Input: part model. Units: mm. Frame: model coordinates. A direction names the side the tool comes from. Round coordinates to 2 decimals unless told otherwise and drop trailing zeros. Write each loop counter-clockwise with the first axis right and the second up, starting at its lowest first coordinate (ties: lowest second). Pieces come first, ordered by that corner, then holes. Notation, with made-up numbers: M 22.5,-21 L 44.5,-21 A14 ccw 44.5,-13 Z; hole C 29,89.5 d7. An arc over 180 degrees is marked long. Use one line per item in the form item = value. Start each with the question number.
Autodesk Inventor part; units mm, degrees
ref_plane "YZ Plane" through (0, 0, 0) normal (1, 0, 0) x (0, 1, 0)
ref_plane "XZ Plane" through (0, 0, 0) normal (0, 1, 0) x (-1, 0, 0)
ref_plane "XY Plane" through (0, 0, 0) normal (0, 0, 1) x (1, 0, 0)
sketch "Sketch1" plane through (0, 0, 0) normal (1, 0, 0) x (0, 1, 0)
  line L0 (0, 0) -> (-165.1, 0) construction
  line L1 (-165.1, 0) -> (-165.1, 152.4) construction
  line L2 (-165.1, 152.4) -> (0, 152.4) construction
  line L3 (0, 152.4) -> (0, 0) construction
  line L4 (0, 152.4) -> (-38.1, 152.4)
  line L5 (-165.1, 0) -> (-165.1, 38.1)
  line L6 (-165.1, 38.1) -> (-38.1, 152.4)
  line L7 (0, 152.4) -> (0, 0)
  line L8 (0, 0) -> (-165.1, 0)
  dimension "d0" = 165.1
  dimension "d1" = 152.4
  dimension "d2" = 38.1
  dimension "d3" = 38.1
extrude "Extrusion1" add sketch "Sketch1" along normal blind 6.35
sketch "Sketch2" plane through (0, 0, 0) normal (-1, 0, 0) x (0, 0, 1)
  line L0 (0, -165.1) -> (0, 0)
  line L1 (38.1, -165.1) -> (0, -165.1)
  point P0 (25.4, -139.7)
  point P1 (25.4, -88.9)
  point P2 (25.4, -38.1)
  dimension "d6" = 25.4
  dimension "d7" = 25.4
  dimension "d8" = 25.4
  dimension "d9" = 25.4
  dimension "d10" = 50.8
  dimension "d11" = 50.8
hole "Hole1" at (0, -139.7, 25.4) at (0, -88.9, 25.4) at (0, -38.1, 25.4) direction (1, 0, 0) diameter 6.35 end through all
sketch "Sketch3" plane through (0, 0, 0) normal (-1, 0, 0) x (0, 0, 1)
  line L0 (0, -165.1) -> (0, 0)
  line L1 (0, 0) -> (25.4, 0)
  line L2 (0, 0) -> (152.4, 0)
  line L3 (25.4, 0) -> (0, -25.4)
  line L4 (0, -165.1) -> (0, 0)
  line L5 (0, -25.4) -> (0, 0)
  dimension "d19" = 25.4
  dimension "d20" = 45
extrude "Extrusion2" cut sketch "Sketch3" against normal blind 6.35
sketch "Sketch4" plane through (0, 0, 0) normal (-1, 0, 0) x (0, 0, 1)
  line L0 (152.4, 0) -> (152.4, -38.1)
  line L1 (25.4, 0) -> (152.4, 0)
  point P0 (0, 0)
  point P1 (139.7, -12.7)
  point P2 (127, -25.4)
  point P3 (114.3, -12.7)
  point P4 (101.6, -25.4)
  dimension "d23" = 12.7
  dimension "d24" = 12.7
  dimension "d25" = 25.4
  dimension "d26" = 25.4
  dimension "d27" = 12.7
  dimension "d28" = 38.1
  dimension "d29" = 50.8
  dimension "d30" = 25.4
hole "Hole2" at (0, -12.7, 139.7) at (0, -25.4, 127) at (0, -12.7, 114.3) at (0, -25.4, 101.6) direction (1, 0, 0) diameter 6.35 end through all
sketch "Sketch5" plane through (0, 0, 0) normal (-1, 0, 0) x (0, 0, 1)
  line L0 (0, -165.1) -> (0, -25.4)
  line L1 (25.4, 0) -> (152.4, 0)
  circle A0 centre (69.85, -19.05) radius 4.7625
  circle A1 centre (52.3875, -25.4) radius 3.175
  circle A2 centre (52.3875, -9.525) radius 3.175
  point P0 (0, 0)
  dimension "d38" = 52.3875
  dimension "d39" = 52.3875
  dimension "d40" = 69.85
  dimension "d41" = 19.05
  dimension "d42" = 9.525
  dimension "d43" = 25.4
  dimension "d44" = 9.525
  dimension "d45" = 6.35
  dimension "d46" = 6.35
extrude "Extrusion3" cut sketch "Sketch5" against normal blind 6.35
sketch "Sketch6" plane through (0, 0, 0) normal (-1, 0, 0) x (0, 0, 1)
  circle A0 centre (52.3875, -9.525) radius 3.175
  circle A1 centre (52.3875, -25.4) radius 3.175
  circle A2 centre (69.85, -19.05) radius 4.7625
  circle A3 centre (114.3, -12.7) radius 3.175
  circle A4 centre (139.7, -12.7) radius 3.175
  circle A5 centre (127, -25.4) radius 3.175
  circle A6 centre (101.6, -25.4) radius 3.175
  line L0 (25.4, 0) -> (0, -25.4)
  line L1 (0, -165.1) -> (0, -25.4)
  line L2 (38.1, -165.1) -> (0, -165.1)
  line L3 (152.4, -38.1) -> (38.1, -165.1)
  line L4 (152.4, 0) -> (152.4, -38.1)
  line L5 (25.4, 0) -> (152.4, 0)
  circle A7 centre (25.4, -38.1) radius 3.175
  circle A8 centre (25.4, -139.7) radius 3.175
  circle A9 centre (25.4, -88.9) radius 3.175
  line L6 (101.8193, -44.45) -> (49.2125, -44.45)
  line L7 (44.45, -49.2125) -> (44.45, -107.6645)
  line L8 (52.7524, -110.8504) -> (105.3592, -52.3984)
  line L9 (152.4, -38.1) -> (38.1, -38.1) construction
  line L10 (38.1, -38.1) -> (38.1, -165.1) construction
  line L11 (38.1, -165.1) -> (152.4, -165.1) construction
  line L12 (152.4, -165.1) -> (152.4, -38.1) construction
  arc A10 (105.3592, -52.3984) -> (101.8193, -44.45) centre (101.8193, -49.2125) ccw
  arc A11 (49.2125, -44.45) -> (44.45, -49.2125) centre (49.2125, -49.2125) ccw
  arc A12 (44.45, -107.6645) -> (52.7524, -110.8504) centre (49.2125, -107.6645) ccw
  point P0 (0, 0)
  dimension "d49" = 6.35
  dimension "d50" = 6.35
  dimension "d52" = 25.4
  dimension "d53" = 4.7625
extrude "Extrusion4" cut sketch "Sketch6" against normal blind 25.4 contours A10 L8 A12 L7 A11 L6
properties part number "mounting bracket" material "Aluminum 6061"
Item 1: First-contact query: pin 1 (5.5 mm diameter, centred on y = -25.4, z = 127, fed in from +X); pin 2 (3 mm diameter, centred on x = 4, y = -43, fed in from -Z); pin 3 (1.9 mm diameter, centred on x = 4, y = -78.5, fed in from +Z) (3 decimals). Flat tips, straight axial feed; report the tip coordinate or a pass-through.
Item 2: Ray query, line 1 (Y direction, x = 1, z = 50.5); line 2 (Z direction, x = 2.5, y = -88.9) (3 decimals); line 3 (Y direction, x = 2.75, z = 25.4) (3 decimals). Return the intervals inside material, ascending. Write a range as from..to.
Item 3: Reachability of faces 4 (the face through (3, -19, 152.4)), 5 (the face through (3, -44.45, 76)) from +Z, -Z, +X, -X, +Y, -Y: full face, straight path, thin tool, end or side. Return the list, or none.
Item 4: Draft query along Y for faces 1 (the face through (3.13, -112.08, 47.43)), 2 (the face through (3, -165.1, 19)), 3 (the face through (3.1, -12.5, 12.9)). Return one class per face: +Y half, -Y half, draft (parallel to the pull), parting line (faces both ways), or undercut.
Item 5: Cut plane A-A (y = -19.05). Output: boundary loops of the cut face in (x, z), plus the area to 3 significant figures.
Item 6: Cut plane C-C (z = 139.7). Output: boundary loops of the cut face in (x, y) (3 decimals).
Item 7: Cut plane D-D (y = -88.9). Output: boundary loops of the cut face in (x, z) (3 decimals).
Item 8: Cut plane B-B (x = 2.5). Give the number of separate pieces and of enclosed holes in the cut face, plus the area to 3 significant figures.
Final values:
q1.pin_1 = through
q1.pin_2 = 0
q1.pin_3 = 116.895
q2.line_1 = -151.32..-112.25, -44.45..-27.95, -22.85..-12.08, -6.97..0
q2.line_2 = 0..22.225, 28.575..44.45, 72.508..106.68
q2.line_3 = -165.1..-142.875, -136.525..-92.075, -85.725..-41.275, -34.925..0
q3.face_4 = +Z, +X, -X, +Y, -Y
q3.face_5 = +X, -X
q4.face_1 = undercut
q4.face_2 = -Y half
q4.face_3 = +Y half
q5.outline = M 0,6.35 L 6.35,6.35 L 6.35,65.09 L 0,65.09 Z; M 0,74.61 L 6.35,74.61 L 6.35,152.4 L 0,152.4 Z
q5.area = 867 mm^2
q6.outline = M 0,-52.211 L 6.35,-52.211 L 6.35,-15.875 L 0,-15.875 Z; M 0,-9.525 L 6.35,-9.525 L 6.35,0 L 0,0 Z
q7.outline = M 0,0 L 6.35,0 L 6.35,22.225 L 0,22.225 Z; M 0,28.575 L 6.35,28.575 L 6.35,44.45 L 0,44.45 Z; M 0,72.508 L 6.35,72.508 L 6.35,106.68 L 0,106.68 Z
q8.separate_pieces = 1
q8.enclosed_holes = 11
q8.area = 14,700 mm^2
